from build123d import *
from build123d import SkipClean  # not in build123d's __all__

# Parameters (mm, degrees)
F1_DEPTH = 3.175


with BuildPart() as f1:
    # F0 (on Top) → F1 (new body, symmetric)
    with BuildSketch(Plane.XY):
        with BuildLine():
            ThreePointArc((0, -77.28), (4, -81.28), (0, -85.28))
            Line((0, -85.28), (0, -89.8525))
            ThreePointArc((0, -89.8525), (6.5348908987, -86.8282391073), (8.4589413231, -79.8892922874))
            Line((8.4589413231, -79.8892922874), (6.35, -67.061714828))
            Line((6.35, -67.061714828), (6.35, 0))
            Line((6.35, 0), (0, 0))
            Line((0, 0), (0, -77.28))
        make_face()
    extrude(amount=F1_DEPTH, both=True)

    # F2: F1 across plane


with BuildPart() as f1_1:
    add(f1.part, clean=False)
    with SkipClean():  # cleaning this boolean's faces spoils the solid; the shape is the same uncleaned
        add(f1.part.mirror(Plane.YZ), clean=False)

    # F3: F1 across plane


with BuildPart() as f1_2:
    add(f1_1.part, clean=False)
    add(f1_1.part.mirror(Plane.XZ), clean=False)


solid = f1_2.part
For this review, take the finished solid that the model builds, in its own axes (mm). A direction names the side the tool comes from. Give positions to 0.01 mm unless a question says otherwise; leave off trailing zeros. Loops run counter-clockwise (first coordinate to the right, second up) from the corner with the lowest first, then second, coordinate; pieces in that order, holes last.
Item 1: Insertion check: pin 1 (1.9 mm diameter, centred on y = 21, z = 0.5, fed in from -X); pin 2 (1.5 mm diameter, centred on y = -3, z = -0.5, fed in from +X); pin 3 (3 mm diameter, centred on x = -2, z = 0.5, fed in from -Y). Each pin has a flat end and moves straight along its axis. Give the tip position at first contact, or say it passes through.
Item 2: Tool access review of faces 1 (the flat face through (7.42, -73.57, 0.04)), 2 (the flat face through (-7.42, -73.57, 0.04)): name each direction out of +Z, -Z, +X, -X, +Y, -Y from which nothing blocks a thin tool from reaching the whole face with its end or side.
Item 3: For line 1 along Y through (x, z) = (0, -0.5); line 2 along Y through (x, z) = (1.25, 0.75); line 3 along X through (y, z) = (26, 0.5), list the stretches that pass through material, from the lowest coordinate up.
Item 4: Take a section at B-B, the plane y = -42.5. State the section outline as (x, z) points (3 decimals).
Item 5: Take a section at A-A, the plane z = -1.5. Give the number of separate pieces and of enclosed holes in the cut face, and give its area (3 significant figures).
Calculated:
1. pin 1: stops at x = -6.35
1. pin 2: stops at x = 6.35
1. pin 3: stops at y = -89.84
2. face 1: +Z, -Z, +X
2. face 2: +Z, -Z, -X
3. line 1: y = -89.85 to -85.28, -77.28 to 77.28, 85.28 to 89.85
3. line 2: y = -89.76 to -85.08, -77.48 to 77.48, 85.08 to 89.76
3. line 3: x = -6.35 to 6.35
4. outline: (-6.35, -3.175) - (6.35, -3.175) - (6.35, 3.175) - (-6.35, 3.175) - close
5. separate pieces: 1
5. enclosed holes: 2
5. area: 2,260 mm2
